Input: part model. Units: mm. Frame: model coordinates. Face numbers are marked on the shaded views. Give positions to 0.01 mm unless a question says otherwise; leave off trailing zeros. Write each loop counter-clockwise with the first axis right and the second up, starting at its lowest first coordinate (ties: lowest second). Pieces come first, ordered by that corner, then holes. Notation, with made-up numbers: (62, 3.5) -> (81, 3.5) arc R8 ccw to (81, 12.5) -> close; hole circle Ø9 at (-27.5, 69). An arc over 180 degrees is marked (long way). Return JSON: item names as keys, results as strings. Group by question number.
Item 1: Section A-A, the plane y = 19. Return loops of the section in (x, z).
Item 2: Section C-C, the plane x = 13. Return loops of the section in (y, z).
Item 3: Section D-D, the plane y = 26. Return loops of the section in (x, z).
Item 4: Mould query, pull axis X, two halves, no side actions, for the marked faces 1, 2, 3 and 4. Classes: released by +X, released by -X, zero draft, split by the parting line, or undercut.
Item 5: Line query: line 1 (Y direction, x = 23, z = -0.5); line 2 (Y direction, x = 23, z = 4); line 3 (X direction, y = 19, z = -2). Output: solid intervals per line, ascending. Write a range as [from, to].
Item 6: Pin query (flat end, axial travel): P1, Ø1.6, axis at y = 1.5, z = 0.5, coming from the +X side; P2, Ø3, axis at x = 37, z = 5, coming from the -Y side; P3, Ø2, axis at x = 18, z = 0.5, coming from the -Y side; P4, Ø0.8, axis at x = 17.5, y = 34.5, coming from the +Z side. Return the tip coordinate at first contact, or that it passes through.
Item 7: Section B-B, the plane z = -3.25. Return loops of the section in (x, y), then the cut area to 3 significant figures.
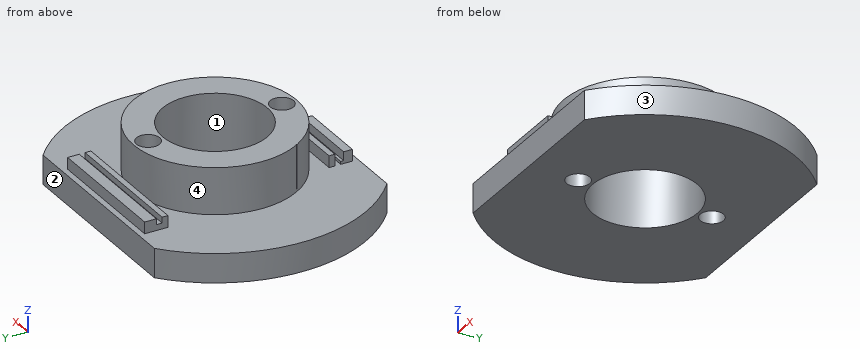
from build123d import *

# Parameters (mm, degrees)
CYLINDER004_R             = 2
CYLINDER004_DEPTH         = 22
CYLINDER005_R             = 2
CYLINDER005_DEPTH         = 22
BOX009_W                  = 46
BOX009_H                  = 10
BOX009_DEPTH              = 10
BOX007_W                  = 46
BOX007_H                  = 10
BOX007_DEPTH              = 10
BOX008_W                  = 54
BOX008_H                  = 53
BOX008_DEPTH              = 15
BOX002_W                  = 5
BOX002_H                  = 10
BOX002_DEPTH              = 13
BOX001_W                  = 23
BOX001_H                  = 1
BOX001_DEPTH              = 13
BOX_W                     = 25
BOX_H                     = 1
BOX_DEPTH                 = 14
BOX003_W                  = 38
BOX003_H                  = 1
BOX003_DEPTH              = 12
BOX004_W                  = 34
BOX004_H                  = 1
BOX004_DEPTH              = 10
FUSION001_PLACEMENT_ANGLE = 180
CYLINDER_R                = 9
CYLINDER_DEPTH            = 28
CYLINDER002_R             = 26
CYLINDER002_DEPTH         = 5
CYLINDER001_R             = 14
CYLINDER001_DEPTH         = 14
CYLINDER003_R             = 26
CYLINDER003_DEPTH         = 5
BOX005_W                  = 23
BOX005_H                  = 4
BOX005_DEPTH              = 2
BOX006_W                  = 12
BOX006_H                  = 4
BOX006_DEPTH              = 2


with BuildPart() as cilindro004:
    # Cylinder004 → Cylinder004 (new body)
    with BuildSketch(Plane(origin=(23, 7.5, -10), x_dir=(1, 0, 0), z_dir=(0, 0, 1))):
        Circle(CYLINDER004_R)
    extrude(amount=CYLINDER004_DEPTH)


with BuildPart() as cilindro005:
    # Cylinder005 → Cylinder005 (new body)
    with BuildSketch(Plane(origin=(23, 30.5, -10), x_dir=(1, 0, 0), z_dir=(0, 0, 1))):
        Circle(CYLINDER005_R)
    extrude(amount=CYLINDER005_DEPTH)


with BuildPart() as cubo009:
    # Box009 → Box009 (new body)
    with BuildSketch(Plane(origin=(0, 39, -6), x_dir=(1, 0, 0), z_dir=(0, 0, 1))):
        with Locations((23, 5)):
            Rectangle(BOX009_W, BOX009_H)
    extrude(amount=BOX009_DEPTH)


with BuildPart() as cubo007:
    # Box007 → Box007 (new body)
    with BuildSketch(Plane(origin=(0, -11, -6), x_dir=(1, 0, 0), z_dir=(0, 0, 1))):
        with Locations((23, 5)):
            Rectangle(BOX007_W, BOX007_H)
    extrude(amount=BOX007_DEPTH)


with BuildPart() as cubo008:
    # Box008 → Box008 (new body)
    with BuildSketch(Plane(origin=(-4, -8, 8), x_dir=(1, 0, 0), z_dir=(0, 0, 1))):
        with Locations((27, 26.5)):
            Rectangle(BOX008_W, BOX008_H)
    extrude(amount=BOX008_DEPTH)


with BuildPart() as cubo002:
    # Box002 → Box002 (new body)
    with BuildSketch(Plane(origin=(1, 0, 0.5), x_dir=(1, 0, 0), z_dir=(0, 0, 1))):
        with Locations((2.5, 5)):
            Rectangle(BOX002_W, BOX002_H)
    extrude(amount=BOX002_DEPTH)


with BuildPart() as cubo001:
    # Box001 → Box001 (new body)
    with BuildSketch(Plane(origin=(0.5, -0.5, 0.5), x_dir=(1, 0, 0), z_dir=(0, 0, 1))):
        with Locations((11.5, 0.5)):
            Rectangle(BOX001_W, BOX001_H)
    extrude(amount=BOX001_DEPTH)


with BuildPart() as fusion:
    # Box → Box (new body)
    with BuildSketch(Plane.XY):
        with Locations((12.5, 0.5)):
            Rectangle(BOX_W, BOX_H)
    extrude(amount=BOX_DEPTH)

    # Fusion: union Cubo002, Cubo001
    add(cubo002.part)
    add(cubo001.part)


with BuildPart() as fusion_1:
    # Fusion placement: moved
    add(fusion.part.moved(Location((5, 2, 0))))


with BuildPart() as cubo003:
    # Box003 → Box003 (new body)
    with BuildSketch(Plane.XY):
        with Locations((19, 0.5)):
            Rectangle(BOX003_W, BOX003_H)
    extrude(amount=BOX003_DEPTH)


with BuildPart() as display:
    # Box004 → Box004 (new body)
    with BuildSketch(Plane(origin=(3, -0.5, 1), x_dir=(1, 0, 0), z_dir=(0, 0, 1))):
        with Locations((17, 0.5)):
            Rectangle(BOX004_W, BOX004_H)
    extrude(amount=BOX004_DEPTH)

    # Fusion001: union Cubo003
    add(cubo003.part)


with BuildPart() as display_1:
    # Fusion001 placement: moved
    add(display.part.moved(Location((4, 36, 13))).rotate(Axis((4, 36, 13), (1, 0, 0)), FUSION001_PLACEMENT_ANGLE))


with BuildPart() as cilindro:
    # Cylinder → Cylinder (new body)
    with BuildSketch(Plane(origin=(23, 19, -7), x_dir=(1, 0, 0), z_dir=(0, 0, 1))):
        Circle(CYLINDER_R)
    extrude(amount=CYLINDER_DEPTH)


with BuildPart() as cilindro002:
    # Cylinder002 → Cylinder002 (new body)
    with BuildSketch(Plane(origin=(23, 19, -5), x_dir=(1, 0, 0), z_dir=(0, 0, 1))):
        Circle(CYLINDER002_R)
    extrude(amount=CYLINDER002_DEPTH)


with BuildPart() as cilindro001:
    # Cylinder001 → Cylinder001 (new body)
    with BuildSketch(Plane(origin=(23, 19, 0), x_dir=(1, 0, 0), z_dir=(0, 0, 1))):
        Circle(CYLINDER001_R)
    extrude(amount=CYLINDER001_DEPTH)


with BuildPart() as cut:
    # Cylinder003 → Cylinder003 (new body)
    with BuildSketch(Plane(origin=(23, 19, 14), x_dir=(1, 0, 0), z_dir=(0, 0, 1))):
        Circle(CYLINDER003_R)
    extrude(amount=CYLINDER003_DEPTH)

    # Fusion002: union Cilindro002, Cilindro001
    add(cilindro002.part)
    add(cilindro001.part)

    # Cut: cut Cilindro
    add(cilindro.part, mode=Mode.SUBTRACT)


with BuildPart() as cut001:
    # Box005 → Box005 (new body)
    with BuildSketch(Plane(origin=(11, 34, 0), x_dir=(1, 0, 0), z_dir=(0, 0, 1))):
        with Locations((11.5, 2)):
            Rectangle(BOX005_W, BOX005_H)
    extrude(amount=BOX005_DEPTH)

    # Fusion003: union Cut
    add(cut.part)

    # Cut001: cut Display
    add(display_1.part, mode=Mode.SUBTRACT)


with BuildPart() as cut007:
    # Box006 → Box006 (new body)
    with BuildSketch(Plane(origin=(15, 0, 0), x_dir=(1, 0, 0), z_dir=(0, 0, 1))):
        with Locations((6, 2)):
            Rectangle(BOX006_W, BOX006_H)
    extrude(amount=BOX006_DEPTH)

    # Fusion004: union Cut001
    add(cut001.part)

    # Cut002: cut Fusion
    add(fusion_1.part, mode=Mode.SUBTRACT)

    # Cut003: cut Cubo008
    add(cubo008.part, mode=Mode.SUBTRACT)

    # Cut004: cut Cubo007
    add(cubo007.part, mode=Mode.SUBTRACT)

    # Cut005: cut Cubo009
    add(cubo009.part, mode=Mode.SUBTRACT)

    # Cut006: cut Cilindro005
    add(cilindro005.part, mode=Mode.SUBTRACT)

    # Cut007: cut Cilindro004
    add(cilindro004.part, mode=Mode.SUBTRACT)


solid = cut007.part
Answer below:
{
 "1": {"outline": "(-3, -5) -> (14, -5) -> (14, 8) -> (9, 8) -> (9, 0) -> (-3, 0) -> close; (32, -5) -> (49, -5) -> (49, 0) -> (37, 0) -> (37, 8) -> (32, 8) -> close"},
 "2": {"outline": "(-1, -5) -> (39, -5) -> (39, 0) -> (38, 0) -> (38, 2) -> (36, 2) -> (36, 1) -> (35, 1) -> (35, 2) -> (34, 2) -> (34, 0) -> (28.8, 0) -> (28.8, 8) -> (9.2, 8) -> (9.2, 0) -> (-1, 0) -> close"},
 "3": {"outline": "(-2.04, -5) -> (17.34, -5) -> (17.34, 8) -> (10.88, 8) -> (10.88, 0) -> (-2.04, 0) -> close; (28.66, -5) -> (48.04, -5) -> (48.04, 0) -> (35.12, 0) -> (35.12, 8) -> (28.66, 8) -> close"},
 "4": {"face 1": "undercut", "face 2": "zero draft", "face 3": "released by +X", "face 4": "split by the parting line"},
 "5": {"line 1": "y = [-1, 5.5], [9.5, 10], [28, 28.5], [32.5, 39]", "line 2": "y = [5, 5.5], [9.5, 10], [28, 28.5], [32.5, 33]", "line 3": "x = [-3, 14], [32, 49]"},
 "6": {"P1": "stops at x = 42.78", "P2": "stops at y = 12.7", "P3": "stops at y = -1", "P4": "stops at z = 2"},
 "7": {"outline": "(6.39, -1) -> (39.61, -1) arc R26 ccw to (39.61, 39) -> (6.39, 39) arc R26 ccw to start; hole circle Ø18 at (23, 19); hole circle Ø4 at (23, 7.5); hole circle Ø4 at (23, 30.5)", "area": "1,570 mm2"}
}
